from build123d import *

# Parameters (mm, degrees)
SKETCH1_R           = 3.175
BOSS_EXTRUDE1_DEPTH = 10


with BuildPart() as part:
    # Sketch1 → Boss-Extrude1 (new body)
    with BuildSketch(Plane(origin=(0, 0, 0), x_dir=(1, 0, 0), z_dir=(0, 1, 0))):
        with BuildLine():
            Line((-60, 27.300970874), (60, 27.300970874))
            Line((60, 27.300970874), (75, -2.699029126))
            Line((75, -2.699029126), (75, -36.699029126))
            Line((75, -36.699029126), (60, -66.699029126))
            Line((60, -66.699029126), (30, -66.699029126))
            Line((30, -66.699029126), (14.348655784, -15.327387893))
            ThreePointArc((14.348655784, -15.327387893), (-0.000213283, -4.699029126), (-14.34901862, -15.327473931))
            Line((-14.34901862, -15.327473931), (-30, -66.699029126))
            Line((-30, -66.699029126), (-60, -66.699029126))
            Line((-60, -66.699029126), (-75, -36.699029126))
            Line((-75, -36.699029126), (-75, -2.699029126))
            Line((-75, -2.699029126), (-60, 27.300970874))
        make_face()
        with Locations(Location((-45, -51.699029126, 0), (0, 0, 270))):
            Circle(SKETCH1_R, mode=Mode.SUBTRACT)
        with Locations(Location((0, 12.300970874, 0), (0, 0, 270))):
            Circle(SKETCH1_R, mode=Mode.SUBTRACT)
        with Locations(Location((45, -51.699029126, 0), (0, 0, 270))):
            Circle(SKETCH1_R, mode=Mode.SUBTRACT)
    extrude(amount=BOSS_EXTRUDE1_DEPTH)


solid = part.part
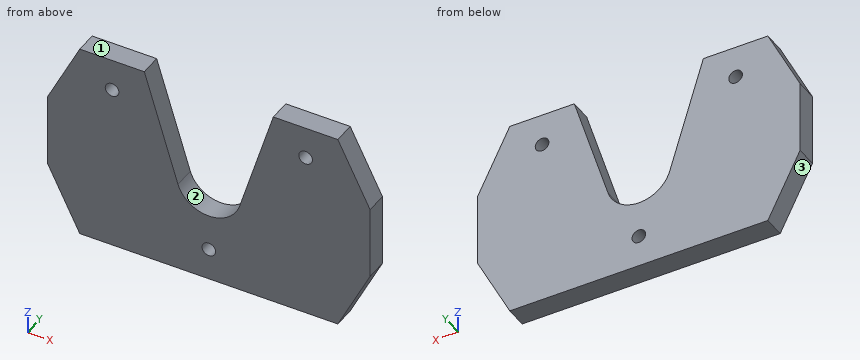
The model under review builds one solid part; all positions refer to its coordinate system, in mm. Face numbers are marked on the shaded views. Coordinates: 2 decimals unless noted, no trailing zeros. Order: outer loops, then holes, each group sorted by start corner. A loop starts at its lowest first (then second) coordinate and runs counter-clockwise, first axis right, second up. Notation, with made-up numbers: (57, 0) -> (97, 0) arc R23 ccw to (97, 27) -> close; hole circle Ø11 at (-36, -9.5). An arc over 180 degrees is marked (long way). Answer in a Markdown table with one row per item.
(1) Consider section C-C (z = 7). Write out the cut boundary in (x, y).
Answers:
| item | result |
|---|---|
| outline | (-75, 0) -> (-7.98, 0) -> (-7.98, 10) -> (-75, 10) -> close; (7.98, 0) -> (75, 0) -> (75, 10) -> (7.98, 10) -> close |
(2) Insertion check: pin 1 (7.5 mm diameter, centred on x = 0, z = -12.3, fed in from +Y); pin 2 (4 mm diameter, centred on x = -45, z = 51.7, fed in from +Y); pin 3 (2 mm diameter, centred on x = 8, y = 5.5, fed in from +Z). Each pin has a flat end and moves straight along its axis. Give the tip position at first contact, or say it passes through.
Answers:
| item | result |
|---|---|
| pin 1 | y = 10 |
| pin 2 | through |
| pin 3 | z = 7.7 |
(3) The part is to be moulded in two halves that separate along X. For the marked faces 1, 2 and 3, say which applies: +X half, -X half, draft (parallel to the pull), parting line (faces both ways), or undercut.
Answers:
| item | result |
|---|---|
| face 1 | draft |
| face 2 | undercut |
| face 3 | -X half |
(4) Consider section D-D (x = -64.5). Write out the cut boundary in (y, z).
Answers:
| item | result |
|---|---|
| outline | (0, -18.3) -> (10, -18.3) -> (10, 57.7) -> (0, 57.7) -> close |
(5) Consider section B-B (y = 3). Write out the cut boundary in (x, z) (3 decimals), plus the area to 3 significant figures.
Answers:
| item | result |
|---|---|
| outline | (-75, 2.699) -> (-60, -27.301) -> (60, -27.301) -> (75, 2.699) -> (75, 36.699) -> (60, 66.699) -> (30, 66.699) -> (14.349, 15.327) arc R15 cw to (-14.349, 15.327) -> (-30, 66.699) -> (-60, 66.699) -> (-75, 36.699) -> close; hole circle Ø6.35 at (-45, 51.699); hole circle Ø6.35 at (0, -12.301); hole circle Ø6.35 at (45, 51.699) |
| area | 10,600 mm² |
(6) Consider section A-A (x = 45). Write out the cut boundary in (y, z), plus the area to 4 significant figures.
Answers:
| item | result |
|---|---|
| outline | (0, -27.3) -> (10, -27.3) -> (10, 48.52) -> (0, 48.52) -> close; (0, 54.87) -> (10, 54.87) -> (10, 66.7) -> (0, 66.7) -> close |
| area | 876.5 mm² |
(7) Wall thickness on line 1 along X through (y, z) = (2.5, 56); line 2 along X through (y, z) = (3.5, 32.5); line 3 along X through (y, z) = (1.75, -5.5): over which ranges is each line inside the solid? List them lowest first.
Answers:
| item | result |
|---|---|
| line 1 | -65.35 to -26.74, 26.74 to 65.35 |
| line 2 | -75 to -19.58, 19.58 to 75 |
| line 3 | -70.9 to 70.9 |
